```python
from build123d import *

# Parameters (mm, degrees)
BOSS_EXTRU_3_DEPTH      = 40
BOSS_EXTRU_3_DEPTH_BACK = 20.027256934
ESQUISSE12_W            = 60
ESQUISSE12_H            = 8
ENL_V_MAT_EXTRU_1_DEPTH = 40
ESQUISSE12_3_W          = 60
ESQUISSE12_3_H          = 13
ENL_V_MAT_EXTRU_2_DEPTH = 40
ESQUISSE20_W            = 0.599721203
ESQUISSE20_H            = 0.763281531
ENL_V_MAT_EXTRU_4_DEPTH = 6
ESQUISSE22_W            = 44
ESQUISSE22_H            = 20
ENL_V_MAT_EXTRU_6_DEPTH = 28
ESQUISSE24_W            = 30
ESQUISSE24_H            = 46.027256934
ESQUISSE24_W_2          = 20
ENL_V_MAT_EXTRU_7_DEPTH = 153
ESQUISSE25_R            = 1
ENL_V_MAT_EXTRU_8_DEPTH = 153
ESQUISSE26_R            = 1
ENL_V_MAT_EXTRU_9_DEPTH = 72


with BuildPart() as part:
    # Esquisse5 → Boss.-Extru.3 (new, two sides: drawn at the far end of the back side and taken through both)
    with BuildSketch(Plane.XY.offset(-BOSS_EXTRU_3_DEPTH_BACK)):
        with BuildLine():
            Line((0, 0), (-150, 0))
            ThreePointArc((-150, 0), (-170, 20), (-150, 40))
            Line((-150, 40), (0, 40))
            ThreePointArc((0, 40), (20, 20), (0, 0))
        make_face()
    extrude(amount=BOSS_EXTRU_3_DEPTH + BOSS_EXTRU_3_DEPTH_BACK)

    # Esquisse12 → Enl_v. mat.-Extru.1 (cut)
    with BuildSketch(Plane(origin=(0, 40, 0), x_dir=(1, 0, 0), z_dir=(0, 1, 0))):
        with Locations((-140, 16.027256934)):
            Rectangle(ESQUISSE12_W, ESQUISSE12_H)
    extrude(amount=-ENL_V_MAT_EXTRU_1_DEPTH, mode=Mode.SUBTRACT)

    # Esquisse12_3 → Enl_v. mat.-Extru.2 (cut)
    with BuildSketch(Plane(origin=(0, 40, 0), x_dir=(1, 0, 0), z_dir=(0, 1, 0))):
        with Locations((-140, -33.5)):
            Rectangle(ESQUISSE12_3_W, ESQUISSE12_3_H)
    extrude(amount=-ENL_V_MAT_EXTRU_2_DEPTH, mode=Mode.SUBTRACT)

    # Esquisse20 → Enl_v. mat.-Extru.4 (cut)
    with BuildSketch(Plane.XY.offset(40)):
        with Locations((-85.88772133, 22.969257081)):
            Rectangle(ESQUISSE20_W, ESQUISSE20_H)
    extrude(amount=-ENL_V_MAT_EXTRU_4_DEPTH, mode=Mode.SUBTRACT)

    # Esquisse22 → Enl_v. mat.-Extru.6 (cut)
    with BuildSketch(Plane(origin=(0, 0, -12.027256934), x_dir=(-1, 0, 0), z_dir=(0, 0, -1))):
        with Locations((142, 20)):
            Rectangle(ESQUISSE22_W, ESQUISSE22_H)
    extrude(amount=-ENL_V_MAT_EXTRU_6_DEPTH, mode=Mode.SUBTRACT)

    # Esquisse24 → Enl_v. mat.-Extru.7 (cut)
    with BuildSketch(Plane(origin=(0, 40, 0), x_dir=(1, 0, 0), z_dir=(0, 1, 0))):
        with Locations((-15, -9.986371533)):
            Rectangle(ESQUISSE24_W, ESQUISSE24_H)
        with Locations((10, -9.986371533)):
            Rectangle(ESQUISSE24_W_2, ESQUISSE24_H)
    extrude(amount=-ENL_V_MAT_EXTRU_7_DEPTH, mode=Mode.SUBTRACT)

    # Esquisse25 → Enl_v. mat.-Extru.8 (cut)
    with BuildSketch(Plane.XY.offset(40)):
        with Locations((0, 20)):
            Circle(ESQUISSE25_R)
    extrude(amount=-ENL_V_MAT_EXTRU_8_DEPTH, mode=Mode.SUBTRACT)

    # Esquisse26 → Enl_v. mat.-Extru.9 (cut)
    with BuildSketch(Plane.XY.offset(27)):
        with Locations((-150, 20)):
            Circle(ESQUISSE26_R)
    extrude(amount=-ENL_V_MAT_EXTRU_9_DEPTH, mode=Mode.SUBTRACT)


solid = part.part
```
Build history of the part. All positions in model axes, mm. A direction names the side the tool comes from. Give positions to 0.01 mm unless a question says otherwise; leave off trailing zeros. Order: outer loops, then holes, each group sorted by start corner. A loop starts at its lowest first (then second) coordinate and runs counter-clockwise, first axis right, second up. Notation, with made-up numbers: M 66,42.25 L 91,42.25 A30 ccw 91,73.25 Z; hole C 59,15 d7. An arc over 180 degrees is marked long. Return JSON: item names as keys, results as strings.
Q1. Two-plate mould, pull along X, no slides. Class faces 1 (the face through (-110, 20, 34)), 2 (the face through (20, 20, -17)), 3 (the face through (-164, 20, 2)): pulls with the +X half, pulls with the -X half, needs draft (parallel to the pull), parting line crosses it, or undercut.
Answer list:
{"face 1": "pulls with the -X half", "face 2": "pulls with the +X half", "face 3": "undercut"}
Q2. 3-axis set-ups, long thin cutter, end or side, ignore diameter. For faces 4 (the face through (-5, 20, -13.027)), 5 (the face through (-140, 20, 27)), 6 (the face through (-110, 20, -16)), 7 (the face through (-120, 20, 2)): which of +Z, -Z, +X, -X, +Y, -Y reach the whole face in a straight line?
Answer list:
{"face 4": "+X, +Y, -Y", "face 5": "+Z, -X, +Y, -Y", "face 6": "-Z, -X, +Y, -Y", "face 7": "-Z"}
Q3. Band-saw the part on C-C (x = -158). Give the cut face in (y, z).
Answer list:
{"outline": "M 1.67,-12.03 L 10,-12.03 L 10,15.97 L 30,15.97 L 30,-12.03 L 38.33,-12.03 L 38.33,27 L 1.67,27 Z"}
Q4. Band-saw the part on A-A (z = -6.5). Give the cut face in (x, y).
Answer list:
{"outline": "M -150,0 L -30,0 L -30,40 L -150,40 A20 ccw Z; hole M -164,10 L -120,10 L -120,30 L -164,30 Z"}
Q5. Band-saw the part on B-B (y = 26). Give the cut face in (x, z), then the cut area to 3 significant figures.
Answer list:
{"outline": "M -169.08,-12.03 L -164,-12.03 L -164,15.97 L -120,15.97 L -120,-12.03 L -110,-12.03 L -110,-20.03 L 19.08,-20.03 L 19.08,-13.03 L -30,-13.03 L -30,33 L 19.08,33 L 19.08,40 L -110,40 L -110,27 L -169.08,27 Z", "area": "6,560 mm^2"}
Q6. Wall check: probe 1 along X at (y, z) = (19, -8); probe 2 along Y at (x, z) = (-150, 20.75); probe 3 along Z at (x, y) = (-7.5, 24). Give the ranges that are in metal, low to high. Write a range as from..to.
Answer list:
{"probe 1": "x = -169.97..-164, -120..-30", "probe 2": "y = 0..19, 21..40", "probe 3": "z = -20.03..-13.03, 33..40"}
Q7. Flat gauge pins, fed straight in: pin 1 (12 mm diameter, centred on y = 16.5, z = -4, fed in from +X); pin 2 (6 mm diameter, centred on y = 28, z = 31.5, fed in from -X); pin 3 (12 mm diameter, centred on x = -144, y = 24.5, fed in from +Z). Where does each tip first touch, or does it go through?
Answer list:
{"pin 1": "stops at x = -30", "pin 2": "stops at x = -110", "pin 3": "stops at z = 27"}
Q8. Band-saw the part on D-D (y = 36.5). Give the cut face in (x, z).
Answer list:
{"outline": "M -161.3,-12.03 L -110,-12.03 L -110,-20.03 L 11.3,-20.03 L 11.3,-13.03 L -30,-13.03 L -30,33 L 11.3,33 L 11.3,40 L -110,40 L -110,27 L -161.3,27 Z"}
